Geometry: final body of the model. Coordinates: model frame, mm. Give positions to 0.01 mm unless a question says otherwise; leave off trailing zeros.
```python
from build123d import *

# Parameters (mm, degrees)
F0_W     = 82.1722075343
F0_H     = 100.6745547056
F1_DEPTH = 50.8
F3_D     = 5.1054
F3_DEPTH = 17.145
F3_TIP   = 1.5338169022
F4_R     = 5.08


with BuildPart() as f1:
    # F0 (on Top) → F1 (new body)
    with BuildSketch(Plane.XY):
        with Locations((4.8976801336, 2.1767504513)):
            Rectangle(F0_W, F0_H)
    extrude(amount=F1_DEPTH)

    # F3
    with Locations(Plane.XY.offset(50.8)):
        with Locations((-16.8170183897, 31.6028743982)):
            Hole(F3_D / 2, depth=F3_DEPTH)
            with Locations((0, 0, -(F3_DEPTH + F3_TIP / 2))):  # 118° drill point
                Cone(0, F3_D / 2, F3_TIP, mode=Mode.SUBTRACT)

    # F4
    f4_edges = [f1.edges().sort_by_distance(p)[0] for p in [
        (45.983784, 2.17675, 50.8),
        (-36.188424, 2.17675, 50.8),
    ]]
    fillet(f4_edges, radius=F4_R)


solid = f1.part
```
Q1. Pin query (flat end, axial travel): pin 1 Ø4.5 at (x, y) = (-16.82, 31.6) entering from +Z; pin 2 Ø2 at (x, y) = (-4, -21) entering from -Z. Return the tip coordinate at first contact, or that it passes through.
Q2. Material intervals for probe 1 along X at (y, z) = (31, 39), sorted ascending.
Q3. Mould query, pull axis X, two halves, no side actions, for faces 1 (the face through (4, 52.514, 25)), 2 (the face through (-16.39, 31.74, 32.39)), 3 (the face through (-19.175, 30.625, 42.107)), 4 (the face through (44.46, 2.88, 49.35)). Classes: +X half, -X half, draft (parallel to the pull), parting line (faces both ways), or undercut.
Resolved:
1. pin 1: stops at z = 33.48
1. pin 2: stops at z = 0
2. probe 1: x = -36.19 to -19.3, -14.34 to 45.98
3. face 1: draft
3. face 2: undercut
3. face 3: undercut
3. face 4: +X half
